Part model, mm, in its own coordinate system. A direction names the side the tool comes from. Round coordinates to 2 decimals unless told otherwise and drop trailing zeros. Loops run counter-clockwise (first coordinate to the right, second up) from the corner with the lowest first, then second, coordinate; pieces in that order, holes last. Notation, with made-up numbers: (10, 42.5) - (38, 42.5) arc R23 cw to (38, 56.5) - close; hole circle Ø7 at (20.25, -8). An arc over 180 degrees is marked (long way). Put each result on its own line as item: value.
from build123d import *

# Parameters (mm, degrees)
SKETCH_8_W           = 140
SKETCH_8_H           = 130
EXTRUDE_2_DEPTH      = 100
SKETCH_9_W           = 119.853608507
SKETCH_9_H           = 114.241733861
CUT_EXTRUDE_2_DEPTH  = 90
SKETCH_10_W          = 140
SKETCH_10_H          = 55.45062913
EXTRUDE_3_DEPTH      = 60
SKETCH_11_W          = 119.853608507
SKETCH_11_H          = 52.765862156
CUT_EXTRUDE_3_DEPTH  = 50
SKETCH_12_W          = 60
SKETCH_12_H          = 55.45062913
EXTRUDE_4_DEPTH      = 50
SKETCH_13_W          = 60
SKETCH_13_H          = 55.45062913
EXTRUDE_5_DEPTH      = 50
SKETCH_15_W          = 41.61767962
SKETCH_15_H          = 50
CUT_EXTRUDE_5_DEPTH  = 50
SKETCH_16_W          = 41.61767962
SKETCH_16_H          = 49.940605531
CUT_EXTRUDE_6_DEPTH  = 220
SKETCH_18_W          = 140
SKETCH_18_H          = 100
EXTRUDE_6_DEPTH      = 20
SKETCH_19_W          = 119.853608507
SKETCH_19_H          = 90
CUT_EXTRUDE_7_DEPTH  = 17
CUT_EXTRUDE_8_DEPTH  = 17
SKETCH_29_R          = 5.01352521
SKETCH_29_R_2        = 5.249816441
SKETCH_29_R_3        = 4.93835751
SKETCH_29_R_4        = 5.104719563
SKETCH_29_R_5        = 4.942569228
SKETCH_29_R_6        = 5.218376227
SKETCH_29_R_7        = 5.109275874
SKETCH_29_R_8        = 4.846735289
CUT_EXTRUDE_9_DEPTH  = 17
EXTRUDE_9_DEPTH      = 4
SKETCH_37_W          = 2
SKETCH_37_H          = 96
EXTRUDE_10_DEPTH     = 4
SKETCH_39_W          = 84
SKETCH_39_H          = 94.106669422
CUT_EXTRUDE_10_DEPTH = 4
SKETCH_40_W          = 2.323035316
SKETCH_40_H          = 2.081311216
CUT_EXTRUDE_12_DEPTH = 94
SKETCH_42_W          = 2.095402412
SKETCH_42_H          = 1.958248824
CUT_EXTRUDE_13_DEPTH = 94
SKETCH_43_W          = 9.619264996
SKETCH_43_H          = 8.129833148
EXTRUDE_11_DEPTH     = 135
SKETCH_44_R          = 1.5
CUT_EXTRUDE_14_DEPTH = 40
SKETCH_45_W          = 19.969543159
SKETCH_45_H          = 19.838905337
EXTRUDE_12_DEPTH     = 20
EXTRUDE_13_DEPTH     = 55.5
CUT_EXTRUDE_15_DEPTH = 45
SKETCH_50_W          = 119.853608507
SKETCH_50_H          = 70
EXTRUDE_14_DEPTH     = 90
SKETCH_51_W          = 102.080516597
SKETCH_51_H          = 36.944055187
CUT_EXTRUDE_17_DEPTH = 70
SKETCH_52_W          = 102.571773441
SKETCH_52_H          = 2.896860024
EXTRUDE_16_DEPTH     = 8
SKETCH_54_W          = 65.620335911
SKETCH_54_H          = 1.893330578
CUT_EXTRUDE_18_DEPTH = 4
SKETCH_55_W          = 6.653347609
SKETCH_55_H          = 11.160454054
EXTRUDE_17_DEPTH     = 8
SKETCH_56_W          = 4.450383643
SKETCH_56_H          = 9.96038244
EXTRUDE_18_DEPTH     = 8
SKETCH_57_R          = 1.5
CUT_EXTRUDE_19_DEPTH = 20
SKETCH_58_W          = 17.801534575
SKETCH_58_H          = 15.470381237
CUT_EXTRUDE_21_DEPTH = 45
SKETCH_59_W          = 17.801534575
SKETCH_59_H          = 13.564090588
CUT_EXTRUDE_22_DEPTH = 25
SKETCH_62_W          = 17.801534575
SKETCH_62_H          = 40.082559496
CUT_REVOLVE_1_ANGLE  = 45


with BuildPart() as part:
    # 草图8 → 凸台-拉伸2 (new body)
    with BuildSketch(Plane(origin=(0, 0, 0), x_dir=(1, 0, 0), z_dir=(0, 1, 0))):
        with Locations((1.794871795, 32.423076923)):
            Rectangle(SKETCH_8_W, SKETCH_8_H)
    extrude(amount=EXTRUDE_2_DEPTH)

    # 草图9 → 切除-拉伸2 (cut)
    with BuildSketch(Plane(origin=(0, 100, 0), x_dir=(1, 0, 0), z_dir=(0, 1, 0))):
        with Locations((2.262528015, 32.69030905)):
            Rectangle(SKETCH_9_W, SKETCH_9_H)
    extrude(amount=-CUT_EXTRUDE_2_DEPTH, mode=Mode.SUBTRACT)

    # 草图10 → 凸台-拉伸3 (add)
    with BuildSketch(Plane(origin=(0, 0, -97.423076923), x_dir=(-1, 0, 0), z_dir=(0, 0, -1))):
        with Locations((-1.794871795, 72.274685435)):
            Rectangle(SKETCH_10_W, SKETCH_10_H)
    extrude(amount=EXTRUDE_3_DEPTH)

    # 草图11 → 切除-拉伸3 (cut)
    with BuildSketch(Plane(origin=(0, 100, 0), x_dir=(1, 0, 0), z_dir=(0, 1, 0))):
        with Locations((2.262528015, 116.194107058)):
            Rectangle(SKETCH_11_W, SKETCH_11_H)
    extrude(amount=-CUT_EXTRUDE_3_DEPTH, mode=Mode.SUBTRACT)

    # 草图12 → 凸台-拉伸4 (add)
    with BuildSketch(Plane.ZY.offset(68.205128205)):
        with Locations((-127.423076923, 72.274685435)):
            Rectangle(SKETCH_12_W, SKETCH_12_H)
    extrude(amount=EXTRUDE_4_DEPTH)

    # 草图13 → 凸台-拉伸5 (add)
    with BuildSketch(Plane(origin=(71.794871795, 0, 0), x_dir=(0, 0, -1), z_dir=(1, 0, 0))):
        with Locations((127.423076923, 72.274685435)):
            Rectangle(SKETCH_13_W, SKETCH_13_H)
    extrude(amount=EXTRUDE_5_DEPTH)

    # 草图15 → 切除-拉伸5 (cut)
    with BuildSketch(Plane(origin=(-57.664276238, 0, 0), x_dir=(0, 0, -1), z_dir=(1, 0, 0))):
        with Locations((121.768198326, 75)):
            Rectangle(SKETCH_15_W, SKETCH_15_H)
    extrude(amount=-CUT_EXTRUDE_5_DEPTH, mode=Mode.SUBTRACT)

    # 草图16 → 切除-拉伸6 (cut)
    with BuildSketch(Plane(origin=(-107.664276238, 0, 0), x_dir=(0, 0, -1), z_dir=(1, 0, 0))):
        with Locations((121.768198326, 75.029697235)):
            Rectangle(SKETCH_16_W, SKETCH_16_H)
    extrude(amount=CUT_EXTRUDE_6_DEPTH, mode=Mode.SUBTRACT)

    # 草图18 → 凸台-拉伸6 (add)
    with BuildSketch(Plane.XY.offset(32.576923077)):
        with Locations((1.794871795, 50)):
            Rectangle(SKETCH_18_W, SKETCH_18_H)
    extrude(amount=EXTRUDE_6_DEPTH)

    # 草图19 → 切除-拉伸7 (cut)
    with BuildSketch(Plane(origin=(0, 0, 24.430557881), x_dir=(-1, 0, 0), z_dir=(0, 0, -1))):
        with Locations((-2.262528015, 55)):
            Rectangle(SKETCH_19_W, SKETCH_19_H)
    extrude(amount=-CUT_EXTRUDE_7_DEPTH, mode=Mode.SUBTRACT)

    # 草图20 → 切除-拉伸8 (cut)
    with BuildSketch(Plane.XZ):
        with BuildLine():
            Line((-42.997677053, -75), (-22.997677053, -75))
            ThreePointArc((-22.997677053, -75), (-17.997677053, -80), (-22.997677053, -85))
            Line((-22.997677053, -85), (-42.997677053, -85))
            ThreePointArc((-42.997677053, -85), (-47.997677053, -80), (-42.997677053, -75))
        make_face()
        with BuildLine():
            Line((22.997677053, -85), (42.997677053, -85))
            ThreePointArc((42.997677053, -85), (47.997677053, -80), (42.997677053, -75))
            Line((42.997677053, -75), (22.997677053, -75))
            ThreePointArc((22.997677053, -75), (17.997677053, -80), (22.997677053, -85))
        make_face()
    extrude(amount=-CUT_EXTRUDE_8_DEPTH, mode=Mode.SUBTRACT)

    # 草图29 → 切除-拉伸9 (cut)
    with BuildSketch(Plane.XZ.offset(-44.54937087)):
        with Locations(Location((-93.309871888, -109.657200503, 0), (0, 0, 270))):
            Circle(SKETCH_29_R)
        with Locations(Location((-65.511669659, -109.657200503, 0), (0, 0, 270))):
            Circle(SKETCH_29_R_2)
        with Locations(Location((-38.174617175, -109.525727046, 0), (0, 0, 270))):
            Circle(SKETCH_29_R_3)
        with Locations(Location((-14.155387991, -109.525727046, 0), (0, 0, 270))):
            Circle(SKETCH_29_R_4)
        with Locations(Location((14.155387991, -109.525727046, 0), (0, 0, 270))):
            Circle(SKETCH_29_R_5)
        with Locations(Location((38.174617175, -109.525727046, 0), (0, 0, 270))):
            Circle(SKETCH_29_R_6)
        with Locations(Location((65.511669659, -109.657200503, 0), (0, 0, 270))):
            Circle(SKETCH_29_R_7)
        with Locations(Location((93.309871888, -109.657200503, 0), (0, 0, 270))):
            Circle(SKETCH_29_R_8)
    extrude(amount=-CUT_EXTRUDE_9_DEPTH, mode=Mode.SUBTRACT)

    # 草图17 → 凸台-拉伸9 (add)
    with BuildSketch(Plane(origin=(0, 0, 0), x_dir=(-1, 0, 0), z_dir=(0, -1, 0))):
        Polygon((44.206117019, 0), (44.206117019, -45.225446523), (-43.793882981, -45.225446523), (-43.793882981, 0), (-43.793882981, 50.774553477), (44.206117019, 50.774553477), align=None)
    extrude(amount=EXTRUDE_9_DEPTH)

    # 草图37 → 凸台-拉伸10 (add)
    with BuildSketch(Plane.XZ.offset(4)):
        with Locations((-45.206117019, -2.774553477)):
            Rectangle(SKETCH_37_W, SKETCH_37_H)
        with Locations((44.793882981, -2.774553477)):
            Rectangle(SKETCH_37_W, SKETCH_37_H)
    extrude(amount=-EXTRUDE_10_DEPTH)

    # 草图39 → 切除-拉伸10 (cut)
    with BuildSketch(Plane.XZ.offset(4)):
        with Locations((0, -3.721218766)):
            Rectangle(SKETCH_39_W, SKETCH_39_H)
    extrude(amount=-CUT_EXTRUDE_10_DEPTH, mode=Mode.SUBTRACT)

    # 草图40 → 切除-拉伸12 (cut)
    with BuildSketch(Plane(origin=(0, 0, -50.774553477), x_dir=(-1, 0, 0), z_dir=(0, 0, -1))):
        with Locations((43.161517658, -1.040655608)):
            Rectangle(SKETCH_40_W, SKETCH_40_H)
    extrude(amount=-CUT_EXTRUDE_12_DEPTH, mode=Mode.SUBTRACT)

    # 草图42 → 切除-拉伸13 (cut)
    with BuildSketch(Plane(origin=(0, 0, -50.774553477), x_dir=(-1, 0, 0), z_dir=(0, 0, -1))):
        with Locations((-43.047701206, -0.979124412)):
            Rectangle(SKETCH_42_W, SKETCH_42_H)
    extrude(amount=-CUT_EXTRUDE_13_DEPTH, mode=Mode.SUBTRACT)

    # 草图43 → 凸台-拉伸11 (add)
    with BuildSketch(Plane.XZ):
        with Locations((54.952979828, 21.790363097)):
            Rectangle(SKETCH_43_W, SKETCH_43_H)
    extrude(amount=EXTRUDE_11_DEPTH)

    # 草图44 → 切除-拉伸14 (cut)
    with BuildSketch(Plane(origin=(0, 0, 17.725446523), x_dir=(-1, 0, 0), z_dir=(0, 0, -1))):
        with Locations((-55.095402412, -71)):
            Circle(SKETCH_44_R)
        with Locations((-55.095402412, -127)):
            Circle(SKETCH_44_R)
    extrude(amount=-CUT_EXTRUDE_14_DEPTH, mode=Mode.SUBTRACT)

    # 草图45 → 凸台-拉伸12 (add)
    with BuildSketch(Plane.XZ):
        with Locations((55.778654561, 21.231716271)):
            Rectangle(SKETCH_45_W, SKETCH_45_H)
    extrude(amount=EXTRUDE_12_DEPTH)

    # 草图46 → 凸台-拉伸13 (add)
    with BuildSketch(Plane(origin=(0, 100, 0), x_dir=(1, 0, 0), z_dir=(0, 1, 0))):
        Polygon((-118.205128205, 97.423076923), (-68.205128205, 52.570357533), (-68.205128205, 97.423076923), align=None)
        Polygon((71.794871795, 97.423076923), (71.794871795, 52.570357533), (121.794871795, 97.423076923), align=None)
    extrude(amount=-EXTRUDE_13_DEPTH)

    # 草图47 → 切除-拉伸15 (cut)
    with BuildSketch(Plane(origin=(0, 100, 0), x_dir=(1, 0, 0), z_dir=(0, 1, 0))):
        Polygon((-107.664276238, 100.959358516), (-57.664276238, 57.344666553), (-57.664276238, 100.959358516), align=None)
        Polygon((112.335723762, 100.959358516), (62.189332269, 57.344666553), (62.189332269, 100.959358516), align=None)
    extrude(amount=-CUT_EXTRUDE_15_DEPTH, mode=Mode.SUBTRACT)

    # 草图50 → 凸台-拉伸14 (add)
    with BuildSketch(Plane(origin=(0, 10, 0), x_dir=(1, 0, 0), z_dir=(0, 1, 0))):
        with Locations((2.262528015, -6.430557881)):
            Rectangle(SKETCH_50_W, SKETCH_50_H)
    extrude(amount=EXTRUDE_14_DEPTH)

    # 草图51 → 切除-拉伸17 (cut)
    with BuildSketch(Plane.XY.offset(52.576923077)):
        with Locations((5.343057287, 63.574399949)):
            Rectangle(SKETCH_51_W, SKETCH_51_H)
    extrude(amount=-CUT_EXTRUDE_17_DEPTH, mode=Mode.SUBTRACT)

    # 草图52 → 凸台-拉伸16 (add)
    with BuildSketch(Plane.XZ.offset(-82.046427542)):
        with Locations((5.588685709, 51.128493065)):
            Rectangle(SKETCH_52_W, SKETCH_52_H)
    extrude(amount=EXTRUDE_16_DEPTH)

    # 草图54 → 切除-拉伸18 (cut)
    with BuildSketch(Plane.XZ.offset(4)):
        with Locations((0.307674718, 44.278781234)):
            Rectangle(SKETCH_54_W, SKETCH_54_H)
    extrude(amount=-CUT_EXTRUDE_18_DEPTH, mode=Mode.SUBTRACT)

    # 草图55 → 凸台-拉伸17 (add)
    with BuildSketch(Plane(origin=(0, 0, 17.725446523), x_dir=(-1, 0, 0), z_dir=(0, 0, -1))):
        with Locations((-54.914340612, -127.919346869)):
            Rectangle(SKETCH_55_W, SKETCH_55_H)
    extrude(amount=-EXTRUDE_17_DEPTH)

    # 草图56 → 凸台-拉伸18 (add)
    with BuildSketch(Plane.XY.offset(25.855279671)):
        with Locations((55.093514005, -127.911898971)):
            Rectangle(SKETCH_56_W, SKETCH_56_H)
    extrude(amount=-EXTRUDE_18_DEPTH)

    # 草图57 → 切除-拉伸19 (cut)
    with BuildSketch(Plane(origin=(0, 0, 17.725446523), x_dir=(-1, 0, 0), z_dir=(0, 0, -1))):
        with Locations((-55.095402412, -126)):
            Circle(SKETCH_57_R)
    extrude(amount=-CUT_EXTRUDE_19_DEPTH, mode=Mode.SUBTRACT)

    # 草图58 → 切除-拉伸21 (cut)
    with BuildSketch(Plane.XY.offset(52.576923077)):
        with Locations((27.013712443, 18.31499218)):
            Rectangle(SKETCH_58_W, SKETCH_58_H)
    extrude(amount=-CUT_EXTRUDE_21_DEPTH, mode=Mode.SUBTRACT)

    # 草图59 → 切除-拉伸22 (cut)
    with BuildSketch(Plane.XZ.offset(-26.050182799)):
        with Locations((27.013712443, 14.545045525)):
            Rectangle(SKETCH_59_W, SKETCH_59_H)
    extrude(amount=-CUT_EXTRUDE_22_DEPTH, mode=Mode.SUBTRACT)

    # 草图62 → 切除-旋转1 (revolve, cut)
    with BuildSketch(Plane(origin=(0, 10.579801562, 0), x_dir=(1, 0, 0), z_dir=(0, 1, 0))):
        with Locations((27.013712443, -32.535643329)):
            Rectangle(SKETCH_62_W, SKETCH_62_H)
    revolve(axis=Axis((18.112945155, 10.579801562, 52.576923077), (1, 0, 0)), revolution_arc=CUT_REVOLVE_1_ANGLE, mode=Mode.SUBTRACT)


solid = part.part
1. Probe line 1 along Z through (x, y) = (-8, 79.5); line 2 along X through (y, z) = (56, -126.5); line 3 along X through (y, z) = (-71, 21). List the from-to ranges inside material, lowest first. Write a range as [from, to].
A:
line 1: z = [-157.42, -142.58], [-28.57, -17.42], [49.68, 52.58]
line 2: x = [-118.21, -107.66], [112.34, 121.79]
line 3: x = [50.14, 53.6], [56.6, 59.76]
2. Band-saw the part on C-C (z = -80). List the corners of the cut face in (x, y), plus the area to 3 significant figures.
A:
outline: (-98.78, 44.5) - (-68.21, 44.5) - (-68.21, 0) - (-48, 0) - (-48, 10) - (-57.66, 10) - (-57.66, 55) - (-83.64, 55) - (-83.64, 100) - (-98.78, 100) - close; (-18, 0) - (18, 0) - (18, 10) - (-18, 10) - close; (48, 0) - (71.79, 0) - (71.79, 44.5) - (102.37, 44.5) - (102.37, 100) - (88.24, 100) - (88.24, 55) - (62.19, 55) - (62.19, 10) - (48, 10) - close
area: 3,670 mm²
3. Band-saw the part on B-B (x = -52). List the corners of the cut face in (y, z).
A:
outline: (0, -97.42) - (44.55, -97.42) - (44.55, -157.42) - (100, -157.42) - (100, -142.58) - (50, -142.58) - (50, -89.81) - (10, -89.81) - (10, -28.57) - (100, -28.57) - (100, 52.58) - (0, 52.58) - close
4. Band-saw the part on A-A (z = -25). List the corners of the cut face in (x, y).
A:
outline: (-68.21, 0) - (-46.21, 0) - (-46.21, -4) - (-42, -4) - (-42, -2.08) - (-44.32, -2.08) - (-44.32, 0) - (44.1, 0) - (44.1, -1.96) - (42, -1.96) - (42, -4) - (45.79, -4) - (45.79, 0) - (71.79, 0) - (71.79, 100) - (-68.21, 100) - close
5. Tool access for faces 1 (the flat face through (1, 30, -89.811)), 2 (the flat face through (27, 26.05, 45)), 3 (the flat face through (5, 82.046, 17)), 4 (the cylindrical face through (18, 4.9, -79.9)): list every direction of +Z, -Z, +X, -X, +Y, -Y with a clear straight run to the whole face (end or side of a thin tool).
A:
face 1: +Y
face 2: +Z
face 3: none
face 4: +Y, -Y
6. Band-saw the part on D-D (y = -50). List the corners of the cut face in (x, z).
A:
outline: (50.14, 17.73) - (59.76, 17.73) - (59.76, 25.86) - (50.14, 25.86) - close
7. Pin check, flat tips, straight feed: P1, Ø8, axis at x = 19, z = -18, coming from the -Y side; P2, Ø2, axis at x = 43, y = -0.5, coming from the -Z side; P3, Ø10, axis at x = 6, z = -103, coming from the -Y side. Stop position of each tip, or through.
A:
P1: stops at y = 0
P2: stops at z = -97.42
P3: stops at y = 44.55
8. Two-plate mould, pull along Z, no slides. Class faces 5 (the flat face through (56, -10, 31.151)), 6 (the flat face through (1, 100, -22)), 7 (the flat face through (5, 64, -17.423)): pulls with the +Z half, pulls with the -Z half, needs draft (parallel to the pull), parting line crosses it, or undercut.
A:
face 5: pulls with the +Z half
face 6: needs draft
face 7: undercut
